```python
from build123d import *

# Parameters (mm, degrees)
SKETCH4_W           = 106.06440689
SKETCH4_H           = 3
SKETCH4_W_2         = 10
SKETCH4_H_2         = 5
BOSS_EXTRUDE1_DEPTH = 52
SKETCH5_R           = 2.1
CUT_EXTRUDE1_DEPTH  = 52
SKETCH6_R           = 2.1
CUT_EXTRUDE2_DEPTH  = 52
SKETCH7_W           = 16
SKETCH7_H           = 82.35034403
CUT_EXTRUDE4_DEPTH  = 124
BOSS_EXTRUDE2_DEPTH = 18
SKETCH9_R           = 2.1
CUT_EXTRUDE5_DEPTH  = 6
BOSS_EXTRUDE3_DEPTH = 18
SKETCH12_R          = 2.1
CUT_EXTRUDE7_DEPTH  = 11
SKETCH13_W          = 30.758926903
SKETCH13_H          = 118.81058029
CUT_EXTRUDE8_DEPTH  = 134
SKETCH14_W          = 18
SKETCH14_H          = 2
CUT_EXTRUDE9_DEPTH  = 10
BOSS_EXTRUDE4_START = -5
SKETCH15_W          = 18
SKETCH15_H          = 2
SKETCH15_R          = 2.1
BOSS_EXTRUDE4_DEPTH = 5
SKETCH16_R          = 2.1
CUT_EXTRUDE10_DEPTH = 68
SKETCH17_R          = 2.1
BOSS_EXTRUDE5_DEPTH = 3
SKETCH18_R          = 2.1
CUT_EXTRUDE11_DEPTH = 68
SKETCH19_W          = 18
SKETCH19_H          = 0.5
CUT_EXTRUDE12_DEPTH = 68
SKETCH20_W          = 7.887405645
SKETCH20_H          = 8
BOSS_EXTRUDE6_DEPTH = 5
SKETCH21_R          = 2.1
CUT_EXTRUDE13_DEPTH = 10


with BuildPart() as part:
    # Sketch4 → Boss-Extrude1 (new body)
    with BuildSketch(Plane(origin=(0, 0, 0), x_dir=(0, 0, -1), z_dir=(1, 0, 0))):
        with Locations((-20.39261819, 190.914352888)):
            Rectangle(SKETCH4_W, SKETCH4_H)
        Polygon((32.639585255, 189.414352888), (32.639585255, 122.064008858), (32.639585255, 117.064008858), (32.639585255, 110.064008858), (37.639585255, 110.064008858), (37.639585255, 192.414352888), (32.639585255, 192.414352888), align=None)
        with Locations((27.639585255, 119.564008858)):
            Rectangle(SKETCH4_W_2, SKETCH4_H_2)
    extrude(amount=BOSS_EXTRUDE1_DEPTH)

    # Sketch5 → Cut-Extrude1 (cut)
    with BuildSketch(Plane(origin=(0, 122.064008858, 0), x_dir=(1, 0, 0), z_dir=(0, 1, 0))):
        with Locations((6, 27.049585255)):
            Circle(SKETCH5_R)
        with Locations((46, 27.639585255)):
            Circle(SKETCH5_R)
    extrude(amount=-CUT_EXTRUDE1_DEPTH, mode=Mode.SUBTRACT)

    # Sketch6 → Cut-Extrude2 (cut)
    with BuildSketch(Plane(origin=(0, 192.414352888, 0), x_dir=(1, 0, 0), z_dir=(0, 1, 0))):
        with Locations((41, -68.424821635)):
            Circle(SKETCH6_R)
        with Locations((11, -68.424821635)):
            Circle(SKETCH6_R)
    extrude(amount=-CUT_EXTRUDE2_DEPTH, mode=Mode.SUBTRACT)

    # Sketch7 → Cut-Extrude4 (cut)
    with BuildSketch(Plane(origin=(0, 0, -37.639585255), x_dir=(-1, 0, 0), z_dir=(0, 0, -1))):
        with Locations((-26, 151.239180873)):
            Rectangle(SKETCH7_W, SKETCH7_H)
    extrude(amount=-CUT_EXTRUDE4_DEPTH, mode=Mode.SUBTRACT)

    # Sketch8 → Boss-Extrude2 (add)
    with BuildSketch(Plane.ZY):
        with BuildLine():
            Line((-37.639585255, 210.414352888), (-37.639585255, 192.414352888))
            Line((-37.639585255, 192.414352888), (-32.639585255, 192.414352888))
            Line((-32.639585255, 192.414352888), (-32.639585255, 207.414352888))
            Line((-32.639585255, 207.414352888), (-13.639585255, 207.414352888))
            Line((-13.639585255, 207.414352888), (-13.639585255, 192.414352888))
            Line((-13.639585255, 192.414352888), (17.89261819, 192.414352888))
            ThreePointArc((17.89261819, 192.414352888), (0.423706042, 198.431388178), (-13.639585255, 210.414352888))
            Line((-13.639585255, 210.414352888), (-37.639585255, 210.414352888))
        make_face()
    extrude(amount=-BOSS_EXTRUDE2_DEPTH)

    # Sketch9 → Cut-Extrude5 (cut)
    with BuildSketch(Plane(origin=(0, 210.414352888, 0), x_dir=(1, 0, 0), z_dir=(0, 1, 0))):
        with Locations((9, 25.639585255)):
            Circle(SKETCH9_R)
    extrude(amount=-CUT_EXTRUDE5_DEPTH, mode=Mode.SUBTRACT)

    # Sketch11 → Boss-Extrude3 (add)
    with BuildSketch(Plane(origin=(52, 0, 0), x_dir=(0, 0, -1), z_dir=(1, 0, 0))):
        with BuildLine():
            Line((32.639585255, 192.414352888), (37.639585255, 192.414352888))
            Line((37.639585255, 192.414352888), (37.639585255, 210.414352888))
            Line((37.639585255, 210.414352888), (13.639585255, 210.414352888))
            ThreePointArc((13.639585255, 210.414352888), (-0.423706042, 198.431388178), (-17.89261819, 192.414352888))
            Line((-17.89261819, 192.414352888), (13.639585255, 192.414352888))
            Line((13.639585255, 192.414352888), (13.639585255, 207.414352888))
            Line((13.639585255, 207.414352888), (32.639585255, 207.414352888))
            Line((32.639585255, 207.414352888), (32.639585255, 192.414352888))
        make_face()
    extrude(amount=-BOSS_EXTRUDE3_DEPTH)

    # Sketch12 → Cut-Extrude7 (cut)
    with BuildSketch(Plane(origin=(0, 210.414352888, 0), x_dir=(1, 0, 0), z_dir=(0, 1, 0))):
        with Locations((43, 25.639585255)):
            Circle(SKETCH12_R)
    extrude(amount=-CUT_EXTRUDE7_DEPTH, mode=Mode.SUBTRACT)

    # Sketch13 → Cut-Extrude8 (cut)
    with BuildSketch(Plane(origin=(0, 210.414352888, 0), x_dir=(1, 0, 0), z_dir=(0, 1, 0))):
        with Locations((9.143188102, -17.675085242)):
            Rectangle(SKETCH13_W, SKETCH13_H)
    extrude(amount=-CUT_EXTRUDE8_DEPTH, mode=Mode.SUBTRACT)

    # Sketch14 → Cut-Extrude9 (cut)
    with BuildSketch(Plane(origin=(0, 122.064008858, 0), x_dir=(1, 0, 0), z_dir=(0, 1, 0))):
        with Locations((43, 23.639585255)):
            Rectangle(SKETCH14_W, SKETCH14_H)
    extrude(amount=-CUT_EXTRUDE9_DEPTH, mode=Mode.SUBTRACT)

    # Sketch15 → Boss-Extrude4 (add)
    with BuildSketch(Plane(origin=(0, 122.064008858, 0), x_dir=(1, 0, 0), z_dir=(0, 1, 0)).offset(BOSS_EXTRUDE4_START)):
        with Locations((43, 23.639585255)):
            Rectangle(SKETCH15_W, SKETCH15_H)
        with Locations((46, 27.639585255)):
            Circle(SKETCH15_R)
    extrude(amount=BOSS_EXTRUDE4_DEPTH)

    # Sketch16 → Cut-Extrude10 (cut)
    with BuildSketch(Plane(origin=(0, 122.064008858, 0), x_dir=(1, 0, 0), z_dir=(0, 1, 0))):
        with Locations((46, 27.639585255)):
            Circle(SKETCH16_R)
    extrude(amount=-CUT_EXTRUDE10_DEPTH, mode=Mode.SUBTRACT)

    # Sketch17 → Boss-Extrude5 (add)
    with BuildSketch(Plane(origin=(0, 192.414352888, 0), x_dir=(1, 0, 0), z_dir=(0, 1, 0))):
        with Locations((41, -68.424821635)):
            Circle(SKETCH17_R)
    extrude(amount=-BOSS_EXTRUDE5_DEPTH)

    # Sketch18 → Cut-Extrude11 (cut)
    with BuildSketch(Plane(origin=(0, 192.414352888, 0), x_dir=(1, 0, 0), z_dir=(0, 1, 0))):
        with Locations((41, -68.424821635)):
            Circle(SKETCH18_R)
    extrude(amount=-CUT_EXTRUDE11_DEPTH, mode=Mode.SUBTRACT)

    # Sketch19 → Cut-Extrude12 (cut)
    with BuildSketch(Plane(origin=(0, 122.064008858, 0), x_dir=(1, 0, 0), z_dir=(0, 1, 0))):
        with Locations((43, 22.889585255)):
            Rectangle(SKETCH19_W, SKETCH19_H)
    extrude(amount=-CUT_EXTRUDE12_DEPTH, mode=Mode.SUBTRACT)

    # Sketch20 → Boss-Extrude6 (add)
    with BuildSketch(Plane(origin=(0, 122.064008858, 0), x_dir=(1, 0, 0), z_dir=(0, 1, 0))):
        with Locations((45.93127306, 28.865937897)):
            Rectangle(SKETCH20_W, SKETCH20_H)
    extrude(amount=-BOSS_EXTRUDE6_DEPTH)

    # Sketch21 → Cut-Extrude13 (cut)
    with BuildSketch(Plane(origin=(0, 122.064008858, 0), x_dir=(1, 0, 0), z_dir=(0, 1, 0))):
        with Locations((46, 27.639585255)):
            Circle(SKETCH21_R)
    extrude(amount=-CUT_EXTRUDE13_DEPTH, mode=Mode.SUBTRACT)


solid = part.part
```
Part model, mm, in its own coordinate system. A direction names the side the tool comes from. Coordinates: 2 decimals unless noted, no trailing zeros. Order: outer loops, then holes, each group sorted by start corner. A loop starts at its lowest first (then second) coordinate and runs counter-clockwise, first axis right, second up. Notation, with made-up numbers: (87, -16.75) -> (106, -16.75) arc R29 ccw to (106, 16.25) -> close; hole circle Ø4 at (34, 4). An arc over 180 degrees is marked (long way). Put each result on its own line as item: value. Start each with the question number.
(1) Pin check, flat tips, straight feed: pin 1 Ø1 at (x, z) = (37, 50) entering from +Y; pin 2 Ø9 at (x, z) = (42.5, -26) entering from -Y; pin 3 Ø4 at (x, y) = (39, 120) entering from +Z. Stop position of each tip, or through.
(2) Which spindle directions (+Z, -Z, +X, -X, +Y, -Y) get a long thin tool onto all of the face, cutting with end or side? Do faces 1 (the face through (43, 122.064, -28)), 2 (the face through (43, 114, -32.64)), 3 (the face through (43, 207.414, -23)). Say none if no direction does.
(3) Mould opens along Z. For faces 4 (the face through (43, 156, -32.64)), 5 (the face through (46.969, 119.599, -25.777)), 6 (the face through (43, 110.064, -35)) say: pulls with the +Z half, pulls with the -Z half, needs draft (parallel to the pull), parting line crosses it, or undercut.
(4) Band-saw the part on B-B (y = 201). Give the cut face in (x, z).
(5) Band-saw the part on C-C (y = 165). Give the cut face in (x, z), then the cut area to 3 significant figures.
(6) Probe line 1 along Y through (x, z) = (39.25, -26); line 2 along Z through (x, y) = (46, 119.6); line 3 along Y through (x, z) = (40.25, -18). List the from-to ranges inside material, lowest first. Write a range as [from, to].
(7) Band-saw the part on A-A (x = 46.75). Give the cut face in (y, z).
Determined:
1. pin 1: stops at y = 192.41
1. pin 2: stops at y = 117.06
1. pin 3: stops at z = -23.14
2. face 1: +Z, +X, -X
2. face 2: +Z, +X, -X, -Y
2. face 3: +X, -X
3. face 4: pulls with the +Z half
3. face 5: undercut
3. face 6: needs draft
4. outline: (34, -37.64) -> (52, -37.64) -> (52, -32.64) -> (34, -32.64) -> close; (34, -13.64) -> (52, -13.64) -> (52, -3.61) -> (34, -3.61) -> close
5. outline: (34, -37.64) -> (52, -37.64) -> (52, -32.64) -> (34, -32.64) -> close
5. area: 90.0 mm²
6. line 1: y = [117.06, 122.06], [189.41, 192.41], [207.41, 210.41]
6. line 2: z = [-37.64, -29.74], [-25.54, -23.14]
6. line 3: y = [189.41, 192.41], [207.41, 210.41]
7. outline: (110.06, -37.64) -> (210.41, -37.64) -> (210.41, -13.64) arc R49.69 cw to (192.41, 17.89) -> (192.41, 73.42) -> (189.41, 73.42) -> (189.41, -32.64) -> (122.06, -32.64) -> (122.06, -29.6) -> (117.06, -29.6) -> (117.06, -32.64) -> (110.06, -32.64) -> close; (117.06, -25.68) -> (122.06, -25.68) -> (122.06, -23.14) -> (117.06, -23.14) -> close; hole (192.41, -32.64) -> (207.41, -32.64) -> (207.41, -13.64) -> (192.41, -13.64) -> close
